Autodesk Inventor part; units mm, degrees
ref_plane "Plan de construction1" through (-34.1506, 32.18, -34.1506) normal (0, 1, 0) x (0.5, 0, 0.8660254)
ref_plane "YZ Plane" through (0, 0, 0) normal (1, 0, 0) x (0, 1, 0)
ref_plane "XZ Plane" through (0, 0, 0) normal (0, 1, 0) x (-1, 0, 0)
sketch "Esquisse1" plane through (0, 0, 0) normal (0, 1, 0) x (-1, 0, 0)
  circle A0 centre (0, 0) radius 215.2 construction
  line L0 (0, -455.3768) -> (0, 455.3768)
  line L1 (-455.3768, 0) -> (455.3768, 0)
  line L2 (70.7107, -254.5584) -> (254.5584, -70.7107)
  line L3 (254.5584, 70.7107) -> (70.7107, 254.5584)
  line L4 (-70.7107, 254.5584) -> (-254.5584, 70.7107)
  line L5 (-254.5584, -70.7107) -> (-70.7107, -254.5584)
  line L6 (0, -325.2691) -> (0, 325.2691) construction
  line L7 (325.2691, 0) -> (-325.2691, 0) construction
  circle A1 centre (-20, 253.412) radius 4
  circle A2 centre (11, -19.0526) radius 2.5
  circle A3 centre (-11, -19.0526) radius 2.5
  circle A4 centre (-22, 0) radius 2.5
  circle A5 centre (-11, 19.0526) radius 2.5
  circle A6 centre (11, 19.0526) radius 2.5
  circle A7 centre (22, 0) radius 2.5
  circle A8 centre (0, 0) radius 30 construction
  circle A9 centre (0, 0) radius 13 construction
  arc A10 (-254.5584, 70.7107) -> (-254.5584, -70.7107) centre (-183.8478, 0) ccw
  arc A11 (70.7107, 254.5584) -> (-70.7107, 254.5584) centre (0, 183.8478) ccw
  arc A12 (-70.7107, -254.5584) -> (70.7107, -254.5584) centre (0, -183.8478) ccw
  arc A13 (254.5584, -70.7107) -> (254.5584, 70.7107) centre (183.8478, 0) ccw
  circle A14 centre (20, 253.412) radius 4
  circle A15 centre (-20, -253.412) radius 4
  circle A16 centre (20, -253.412) radius 4
  circle A17 centre (-254.2, 0) radius 4
  circle A18 centre (254.2, 0) radius 4
  point P0 (0, 0)
  dimension "d1" = 460
  dimension "d2" = 8
  dimension "d3" = 35
  dimension "d13" = 100
  dimension "d14" = 20
  dimension "d15" = 35
ref_plane "Plan de construction1" through (-34.1506, 32.18, -34.1506) normal (0, 1, 0) x (0.5, 0, 0.8660254)
extrude "Extrusion1" add sketch "Esquisse1" along normal blind 40.5 contours A12 L5 A10 L1 A17 A4 L0 | L0 L1 A7 A18 A13 L2 A12 | L1 A4 A17 A10 L4 A11 L0 | L0 A11 L3 A13 L1 A18 A7
sketch "Esquisse2" plane through (0, 0, 0) normal (1, 0, 0) x (0, 1, 0)
  line L0 (0, 215.2) -> (0, -215.2)
  spline S0 degree 3 poles (0, 200.2) (0, 199.1288) (0.0427, 197.117) (0.1932, 194.8886) (0.4094, 192.844) (0.6322, 191.3431) (0.9669, 189.6041) (1.2775, 188.3098) (1.7156, 186.7818) (2.1051, 185.619) (2.6389, 184.2112) (3.1032, 183.1108) (3.7289, 181.7436) (4.2649, 180.6479) (4.9765, 179.2567) (5.5773, 178.1196) (6.363, 176.6528) (7.017, 175.4374) (7.8605, 173.8529) (8.5535, 172.5284) (9.4365, 170.7907) (10.1537, 169.3309) (11.0581, 167.4098) (11.7859, 165.7925) (12.6956, 163.6626) (13.4217, 161.8692) (14.3225, 159.5092) (15.0362, 157.5244) (15.9156, 154.9177) (16.6075, 152.7301) (17.4542, 149.8647) (18.1158, 147.4666) (18.9197, 144.3355) (19.5431, 141.7234) (20.2945, 138.3249) (20.8724, 135.5001) (21.5631, 131.8402) (22.0894, 128.811) (22.7129, 124.904) (23.1834, 121.6852) (23.7349, 117.5541) (24.1466, 114.1673) (24.6235, 109.8437) (24.9748, 106.3179) (25.3761, 101.842) (25.667, 98.213) (25.9934, 93.6343) (26.2251, 89.945) (26.4792, 85.3215) (26.6546, 81.6221) (26.8408, 77.0209) (26.9641, 73.3685) (27.0885, 68.8656) (27.1653, 65.3246) (27.236, 61.005) (27.2735, 57.6471) (27.3002, 53.6047) (27.307, 50.5086) (27.3014, 46.8466) (27.2875, 44.0985) (27.2632, 40.9295) (27.2402, 38.6236) (27.2152, 36.3262) (27.2005, 34.9709) (27.1891, 33.7716) (27.1821, 32.8731) (27.18, 32.27) (27.18, 32) knots 1 1 1 1 1.041667 1.083333 1.104167 1.145833 1.166667 1.208333 1.229167 1.270833 1.291667 1.333333 1.354167 1.395833 1.416667 1.458333 1.479167 1.520833 1.541667 1.583333 1.604167 1.645833 1.666667 1.708333 1.729167 1.770833 1.791667 1.833333 1.854167 1.895833 1.916667 1.958333 1.979167 2.020833 2.041667 2.083333 2.104167 2.145833 2.166667 2.208333 2.229167 2.270833 2.291667 2.333333 2.354167 2.395833 2.416667 2.458333 2.479167 2.520833 2.541667 2.583333 2.604167 2.645833 2.666667 2.708333 2.729167 2.770833 2.791667 2.833333 2.854167 2.895833 2.916667 2.947917 2.958333 2.979167 3 3 3 3
  line L1 (27.18, 32) -> (27.18, -32)
  line L2 (27.18, 0) -> (0, 0)
  line L3 (-10.4655, 0) -> (47.1338, 0)
  line L4 (0, 215.2) -> (2, 215.2)
  line L5 (2, 215.2) -> (2, 220.2)
  line L6 (2, 220.2) -> (0, 220.2)
  line L7 (0, 220.2) -> (0, 215.2)
  point P0 (0, 200.1682)
  dimension "d11" = 5
  dimension "d12" = 2
revolve "Révolution1" cut sketch "Esquisse2" angle 360 about axis through (0, -10, 0) along (0, 1, 0)
equation "\"d15\" = d3"
properties part number "wheel_rim_mold_A"
The model under review builds one solid part; all positions refer to its coordinate system, in mm. A direction names the side the tool comes from. Give positions to 0.01 mm unless a question says otherwise; leave off trailing zeros. Write each loop counter-clockwise with the first axis right and the second up, starting at its lowest first coordinate (ties: lowest second). Pieces come first, ordered by that corner, then holes.
1. Tool access review of faces 4 (the flat face through (161.35, 19.97, 163.92)), 5 (the flat face through (-211, 2, 48)): name each direction out of +Z, -Z, +X, -X, +Y, -Y from which nothing blocks a thin tool from reaching the whole face with its end or side.
2. Wall thickness on L1, parallel to Z at x = 11, y = 37.5; L2, parallel to Y at x = -166.5, z = 83; L3, parallel to Y at x = -77, z = -106.5: over which ranges is each line inside the solid? List them lowest first.
3. Add section B-B, the plane z = 239.5. Write out the cut boundary in (x, y), plus the area to 3 significant figures.
4. Draft analysis for pull direction X (two halves, no side actions). For faces 1 (the cylindrical face through (283.84, 19.97, -1.1)), 2 (the flat face through (0, 27.18, 0)), 3 (the cylindrical face through (-1.1, 19.97, -283.84)), state which applies: +X half, -X half, draft (parallel to the pull), parting line (faces both ways), or undercut.
5. For P1, Ø5, axis at x = -29, y = 21, coming from the -Z side; P2, Ø6.5, axis at x = 11, z = 19.05, coming from the -Y side; P3, Ø1, axis at x = -200, y = 31.5, coming from the -Z side, all flat-tipped, find the tip position at first contact; note any pin that passes through.
6. Add section A-A, the plane y = 13.5. Count the separate pieces of the cut face and the enclosed holes in it, plus the area to 3 significant figures.
Worked answers:
1. face 4: +Z, +X, +Y, -Y
1. face 5: -Y
2. L1: z = -283.24 to -21.55, -16.55 to 16.55, 21.55 to 283.24
2. L2: y = 1.97 to 40.5
2. L3: y = 21.63 to 40.5
3. outline: (-85.77, 0) - (85.77, 0) - (85.77, 40.5) - (-85.77, 40.5) - close
3. area: 6,950 mm2
4. face 1: +X half
4. face 2: undercut
4. face 3: parting line
5. P1: stops at z = -280.27
5. P2: stops at y = 27.18
5. P3: stops at z = -125.77
6. separate pieces: 1
6. enclosed holes: 7
6. area: 121,000 mm2
